from build123d import *

# Parameters (mm, degrees)
SKETCH_1_R      = 20.75
EXTRUDE_1_DEPTH = 5


with BuildPart() as part:
    # 草图1 → 凸台-拉伸1 (new body)
    with BuildSketch(Plane.XY):
        Circle(SKETCH_1_R)
        with BuildLine():
            ThreePointArc((-12.124355653, 5.5), (-10.624355653, 7), (-12.124355653, 8.5))
            ThreePointArc((-12.124355653, 8.5), (-13.624355653, 7), (-12.124355653, 5.5))
        make_face(mode=Mode.SUBTRACT)
        with BuildLine():
            ThreePointArc((-12.124355653, -8.5), (-10.624355653, -7), (-12.124355653, -5.5))
            ThreePointArc((-12.124355653, -5.5), (-13.624355653, -7), (-12.124355653, -8.5))
        make_face(mode=Mode.SUBTRACT)
        with BuildLine():
            ThreePointArc((0, -15.5), (1.5, -14), (0, -12.5))
            ThreePointArc((0, -12.5), (-1.5, -14), (0, -15.5))
        make_face(mode=Mode.SUBTRACT)
        with BuildLine():
            ThreePointArc((12.124355653, -8.5), (13.624355653, -7), (12.124355653, -5.5))
            ThreePointArc((12.124355653, -5.5), (10.624355653, -7), (12.124355653, -8.5))
        make_face(mode=Mode.SUBTRACT)
        with BuildLine():
            ThreePointArc((12.124355653, 5.5), (13.624355653, 7), (12.124355653, 8.5))
            ThreePointArc((12.124355653, 8.5), (10.624355653, 7), (12.124355653, 5.5))
        make_face(mode=Mode.SUBTRACT)
        with BuildLine():
            ThreePointArc((0, 12.5), (1.5, 14), (0, 15.5))
            ThreePointArc((0, 15.5), (-1.5, 14), (0, 12.5))
        make_face(mode=Mode.SUBTRACT)
        with BuildLine():
            ThreePointArc((10.6, 0), (7.495331881, 7.495331881), (0, 10.6))
            ThreePointArc((0, 10.6), (-7.495331881, 7.495331881), (-10.6, 0))
            ThreePointArc((-10.6, 0), (0, -10.6), (10.6, 0))
        make_face(mode=Mode.SUBTRACT)
    extrude(amount=EXTRUDE_1_DEPTH)


solid = part.part
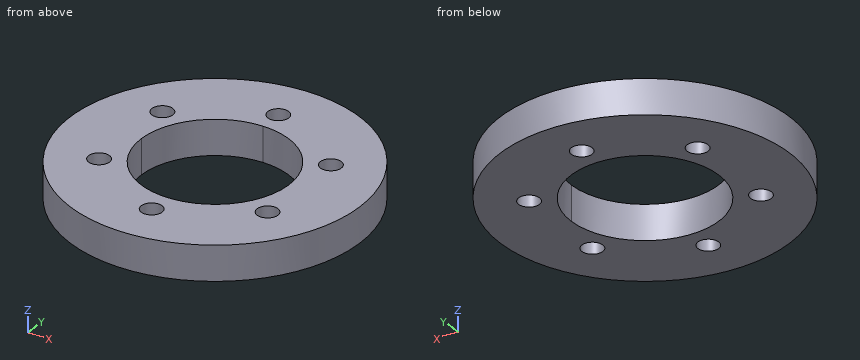
Build history of the part. All positions in model axes, mm. Round coordinates to 2 decimals unless told otherwise and drop trailing zeros. Loops run counter-clockwise (first coordinate to the right, second up) from the corner with the lowest first, then second, coordinate; pieces in that order, holes last. Notation, with made-up numbers: (-1.75, 11.5) -> (15.25, 11.5) arc R29 cw to (15.25, 50.5) -> close; hole circle Ø5 at (89, -21). An arc over 180 degrees is marked (long way). One line per item, written item: value. Start each with the question number.
Q1. Probe line 1 along X through (y, z) = (7, 3.55); line 2 along Y through (x, z) = (-12, 2.3); line 3 along Y through (x, z) = (-11.5, 0.4). List the from-to ranges inside material, lowest first.
Q2. Cut at A-A on x = 5.5. List the corners of the cut face in (y, z).
Q3. Drop flat-ended pins along their axis: pin 1 Ø2 at (x, z) = (-8, 3) entering from -Y; pin 2 Ø1 at (x, z) = (-14.5, 4) entering from +Y; pin 3 Ø1.8 at (x, y) = (-12.12, 7) entering from +Z (3 decimals); pin 4 Ø2 at (x, z) = (12, 2.5) entering from -Y. Give the stop position or say it passes through.
Q4. Cut at D-D on y = -0.5. List the corners of the cut face in (x, z), plus the area to 3 significant figures.
Q5. Cut at C-C on z = 1.1. List the corners of the cut face in (x, y).
Q6. Cut at B-B on y = 7. List the corners of the cut face in (x, z).
Computed:
1. line 1: -19.53 to -13.62, -10.62 to -7.96, 7.96 to 10.62, 13.62 to 19.53
1. line 2: -16.93 to -8.49, -5.51 to 5.51, 8.49 to 16.93
1. line 3: -17.27 to -8.36, -5.64 to 5.64, 8.36 to 17.27
2. outline: (-20.01, 0) -> (-9.06, 0) -> (-9.06, 5) -> (-20.01, 5) -> close; (9.06, 0) -> (20.01, 0) -> (20.01, 5) -> (9.06, 5) -> close
3. pin 1: y = -19.53
3. pin 2: y = 15.32
3. pin 3: through
3. pin 4: y = -17.59
4. outline: (-20.74, 0) -> (-10.59, 0) -> (-10.59, 5) -> (-20.74, 5) -> close; (10.59, 0) -> (20.74, 0) -> (20.74, 5) -> (10.59, 5) -> close
4. area: 102 mm²
5. outline: circle Ø41.5 at (0, 0); hole circle Ø3 at (-12.12, -7); hole circle Ø3 at (-12.12, 7); hole circle Ø21.2 at (0, 0); hole circle Ø3 at (0, -14); hole circle Ø3 at (0, 14); hole circle Ø3 at (12.12, -7); hole circle Ø3 at (12.12, 7)
6. outline: (-19.53, 0) -> (-13.62, 0) -> (-13.62, 5) -> (-19.53, 5) -> close; (-10.62, 0) -> (-7.96, 0) -> (-7.96, 5) -> (-10.62, 5) -> close; (7.96, 0) -> (10.62, 0) -> (10.62, 5) -> (7.96, 5) -> close; (13.62, 0) -> (19.53, 0) -> (19.53, 5) -> (13.62, 5) -> close
